from build123d import *

# Parameters (mm, degrees)
SKETCH_1_W           = 135
SKETCH_1_H           = 80
EXTRUDE_1_DEPTH      = 80
SKETCH_6_W           = 45
SKETCH_6_H           = 80
CUT_EXTRUDE_1_DEPTH  = 35
SKETCH_5_W           = 45
SKETCH_5_H           = 80
CUT_EXTRUDE_2_DEPTH  = 35
SKETCH_7_W           = 80
SKETCH_7_H           = 70
CUT_EXTRUDE_3_DEPTH  = 75
SKETCH_8_W           = 87.8
SKETCH_8_H           = 77.8
SKETCH_8_W_2         = 82.2
SKETCH_8_H_2         = 72.2
CUT_EXTRUDE_4_DEPTH  = 10
SKETCH_9_R           = 5
CUT_EXTRUDE_5_DEPTH  = 32.4
SKETCH_10_W          = 21.5
SKETCH_10_H          = 15
CUT_EXTRUDE_6_DEPTH  = 10
SKETCH_12_W          = 15.816906699
SKETCH_12_H          = 10
CUT_EXTRUDE_7_DEPTH  = 45
CUT_EXTRUDE_8_DEPTH  = 3
SKETCH_15_W          = 10
SKETCH_15_H          = 10
CUT_EXTRUDE_9_DEPTH  = 6
SKETCH_17_R          = 1.095275866
CUT_EXTRUDE_11_DEPTH = 7
SKETCH_18_W          = 5
SKETCH_18_H          = 5
SKETCH_18_R          = 1.1
EXTRUDE_2_DEPTH      = 5


with BuildPart() as part:
    # 草圖1 → 填料-伸長1 (new body)
    with BuildSketch(Plane.XY):
        with Locations((-8.008902174, 5.58988764)):
            Rectangle(SKETCH_1_W, SKETCH_1_H)
    extrude(amount=EXTRUDE_1_DEPTH)

    # 草圖6 → 除料-伸長1 (cut)
    with BuildSketch(Plane(origin=(0, 45.58988764, 0), x_dir=(1, 0, 0), z_dir=(0, 1, 0))):
        with Locations((36.991097826, -40)):
            Rectangle(SKETCH_6_W, SKETCH_6_H)
    extrude(amount=-CUT_EXTRUDE_1_DEPTH, mode=Mode.SUBTRACT)

    # 草圖5 → 除料-伸長2 (cut)
    with BuildSketch(Plane.XZ.offset(34.41011236)):
        with Locations((36.991097826, 40)):
            Rectangle(SKETCH_5_W, SKETCH_5_H)
    extrude(amount=-CUT_EXTRUDE_2_DEPTH, mode=Mode.SUBTRACT)

    # 草圖7 → 除料-伸長3 (cut)
    with BuildSketch(Plane.XY):
        with Locations((-30.508902174, 5.58988764)):
            Rectangle(SKETCH_7_W, SKETCH_7_H)
    extrude(amount=CUT_EXTRUDE_3_DEPTH, mode=Mode.SUBTRACT)

    # 草圖8 → 除料-伸長4 (cut)
    with BuildSketch(Plane(origin=(0, 0, 0), x_dir=(-1, 0, 0), z_dir=(0, 0, -1))):
        with Locations((30.508902174, 5.58988764)):
            Rectangle(SKETCH_8_W, SKETCH_8_H)
        with Locations((30.508902174, 5.58988764)):
            Rectangle(SKETCH_8_W_2, SKETCH_8_H_2, mode=Mode.SUBTRACT)
    extrude(amount=-CUT_EXTRUDE_4_DEPTH, mode=Mode.SUBTRACT)

    # 草圖9 → 除料-伸長5 (cut)
    with BuildSketch(Plane(origin=(14.491097826, 0, 0), x_dir=(0, 0, -1), z_dir=(1, 0, 0))):
        with Locations((-65, 30.58988764)):
            Circle(SKETCH_9_R)
        with Locations((-20, -19.41011236)):
            Circle(SKETCH_9_R)
    extrude(amount=-CUT_EXTRUDE_5_DEPTH, mode=Mode.SUBTRACT)

    # 草圖10 → 除料-伸長6 (cut)
    with BuildSketch(Plane(origin=(0, -34.41011236, 0), x_dir=(-1, 0, 0), z_dir=(0, -1, 0))):
        with Locations((24.758902174, -22.5)):
            Rectangle(SKETCH_10_W, SKETCH_10_H)
    extrude(amount=-CUT_EXTRUDE_6_DEPTH, mode=Mode.SUBTRACT)

    # 草圖12 → 除料-伸長7 (cut)
    with BuildSketch(Plane(origin=(14.491097826, 0, 0), x_dir=(0, 0, -1), z_dir=(1, 0, 0))):
        with Locations((-72.09154665, 5.58988764)):
            Rectangle(SKETCH_12_W, SKETCH_12_H)
        with Locations((-7.90845335, 5.58988764)):
            Rectangle(SKETCH_12_W, SKETCH_12_H)
    extrude(amount=CUT_EXTRUDE_7_DEPTH, mode=Mode.SUBTRACT)

    # 草圖14 → 除料-伸長8 (cut)
    with BuildSketch(Plane(origin=(0, 0.58988764, 0), x_dir=(-1, 0, 0), z_dir=(0, -1, 0))):
        with BuildLine():
            Line((-38.009101008, -35.10282789), (-21.517914827, -38.5))
            ThreePointArc((-21.517914827, -38.5), (-20.017914827, -40), (-21.517914827, -41.5))
            Line((-21.517914827, -41.5), (-38.009101008, -44.89717211))
            ThreePointArc((-38.009101008, -44.89717211), (-39.017914827, -45), (-40.026728646, -44.89717211))
            Line((-40.026728646, -44.89717211), (-56.517914827, -41.5))
            ThreePointArc((-56.517914827, -41.5), (-58.017914827, -40), (-56.517914827, -38.5))
            Line((-56.517914827, -38.5), (-40.026728646, -35.10282789))
            ThreePointArc((-40.026728646, -35.10282789), (-39.017914827, -35), (-38.009101008, -35.10282789))
        make_face()
    extrude(amount=-CUT_EXTRUDE_8_DEPTH, mode=Mode.SUBTRACT)

    # 草圖15 → 除料-伸長9 (cut)
    with BuildSketch(Plane(origin=(0, 10.58988764, 0), x_dir=(1, 0, 0), z_dir=(0, 1, 0))):
        with Locations((39.491097826, -39.816906699)):
            Rectangle(SKETCH_15_W, SKETCH_15_H)
    extrude(amount=-CUT_EXTRUDE_9_DEPTH, mode=Mode.SUBTRACT)

    # 草圖17 → 除料-伸長11 (cut)
    with BuildSketch(Plane(origin=(0, 0.58988764, 0), x_dir=(-1, 0, 0), z_dir=(0, -1, 0))):
        with Locations((-39.017914827, -40)):
            Circle(SKETCH_17_R)
    extrude(amount=-CUT_EXTRUDE_11_DEPTH, mode=Mode.SUBTRACT)

    # 草圖18 → 填料-伸長2 (add)
    with BuildSketch(Plane.XY):
        with Locations((11.991097826, 48.08988764)):
            Rectangle(SKETCH_18_W, SKETCH_18_H)
        with Locations((11.991097826, 48.08988764)):
            Circle(SKETCH_18_R, mode=Mode.SUBTRACT)
        with Locations((-73.008902174, 48.08988764)):
            Rectangle(SKETCH_18_W, SKETCH_18_H)
        with Locations((-73.008902174, 48.08988764)):
            Circle(SKETCH_18_R, mode=Mode.SUBTRACT)
        with Locations((-73.008902174, -36.91011236)):
            Rectangle(SKETCH_18_W, SKETCH_18_H)
        with Locations((-73.008902174, -36.91011236)):
            Circle(SKETCH_18_R, mode=Mode.SUBTRACT)
        with Locations((11.991097826, -36.91011236)):
            Rectangle(SKETCH_18_W, SKETCH_18_H)
        with Locations((11.991097826, -36.91011236)):
            Circle(SKETCH_18_R, mode=Mode.SUBTRACT)
    extrude(amount=EXTRUDE_2_DEPTH)


solid = part.part
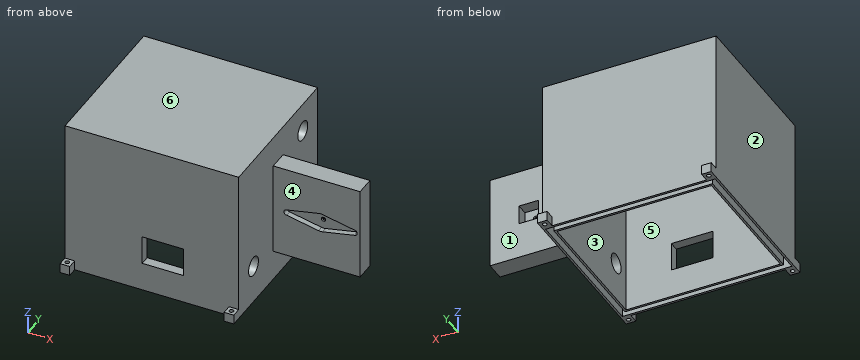
CAD build for the part. Positions are in the model's coordinates, mm. Face numbers are marked on the shaded views. A direction names the side the tool comes from. Round coordinates to 2 decimals unless told otherwise and drop trailing zeros. Order: outer loops, then holes, each group sorted by start corner. A loop starts at its lowest first (then second) coordinate and runs counter-clockwise, first axis right, second up. Notation, with made-up numbers: (-25.5, 57) -> (-17.5, 57) arc R20 ccw to (-17.5, 75) -> close; hole circle Ø8 at (29, 34.25). An arc over 180 degrees is marked (long way). Write item = value, one per line. Start each with the question number.
(1) Cut at D-D, the plane y = 38.5. List the corners of the cut face in (x, z), then the cut area to 3 significant figures.
(2) Cut at C-C, the plane z = 55.5. List the corners of the cut face in (x, y), then the cut area to 3 significant figures.
(3) Pin check, flat tips, straight feed: P1, Ø3.5, axis at x = 11.99, y = 48.09, coming from the -Z side; P2, Ø3, axis at x = -32.5, z = 50.5, coming from the +Y side; P3, Ø4, axis at x = -44.5, y = -25.5, coming from the -Z side; P4, Ø11, axis at x = 43.5, z = 38, coming from the -Y side. Stop position of each tip, or through.
(4) Cut at B-B, the plane z = 20. List the corners of the cut face in (x, y), then the cut area to 3 significant figures.
(5) Probe line 1 (Y direction, x = -70, z = 22); line 2 (X direction, y = -21.5, z = 65); line 3 (X direction, y = -29.5, z = 21). List the from-to ranges inside material, lowest first. Write a range as [from, to].
(6) Which spindle directions (+Z, -Z, +X, -X, +Y, -Y) get a long thin tool onto all of the face, cutting with end or side? Do the marked faces 4, 5 and 6. Say none if no direction does.
(7) Cut at A-A, the plane x = -20.5. List the corners of the cut face in (y, z).
(8) Pull direction Y, two halves, no side cores. Call the marked faces 1, 2 and 3: released by +Y, released by -Y, zero draft, split by the parting line, or undercut.
Model answer:
q1.outline = (-75.51, 0) -> (-74.41, 0) -> (-74.41, 10) -> (-71.61, 10) -> (-71.61, 0) -> (-70.51, 0) -> (-70.51, 75) -> (9.49, 75) -> (9.49, 0) -> (10.59, 0) -> (10.59, 10) -> (13.39, 10) -> (13.39, 0) -> (14.49, 0) -> (14.49, 80) -> (-75.51, 80) -> close
q1.area = 1,140 mm2
q2.outline = (-75.51, -34.41) -> (14.49, -34.41) -> (14.49, 0.59) -> (59.49, 0.59) -> (59.49, 10.59) -> (14.49, 10.59) -> (14.49, 45.59) -> (-75.51, 45.59) -> close; hole (-70.51, -29.41) -> (9.49, -29.41) -> (9.49, 40.59) -> (-70.51, 40.59) -> close
q2.area = 2,050 mm2
q3.P1 = 0
q3.P2 = 45.59
q3.P3 = 75
q3.P4 = 0.59
q4.outline = (-75.51, -34.41) -> (-35.51, -34.41) -> (-35.51, -29.41) -> (-70.51, -29.41) -> (-70.51, 40.59) -> (9.49, 40.59) -> (9.49, -14.41) -> (14.49, -14.41) -> (14.49, 0.59) -> (59.49, 0.59) -> (59.49, 10.59) -> (14.49, 10.59) -> (14.49, 45.59) -> (-75.51, 45.59) -> close; (-14.01, -34.41) -> (14.49, -34.41) -> (14.49, -24.41) -> (9.49, -24.41) -> (9.49, -29.41) -> (-14.01, -29.41) -> close
q4.area = 1,890 mm2
q5.line_1 = [-34.41, -29.41], [40.59, 45.59]
q5.line_2 = [-75.51, -70.51], [9.49, 14.49]
q5.line_3 = [-75.51, -35.51], [-14.01, 14.49]
q6.face_4 = +Z, -Z, +X, -Y
q6.face_5 = -Z
q6.face_6 = +Z, +X, -X, +Y, -Y
q7.outline = (-34.41, 0) -> (-33.31, 0) -> (-33.31, 10) -> (-30.51, 10) -> (-30.51, 0) -> (-29.41, 0) -> (-29.41, 15) -> (-34.41, 15) -> close; (-34.41, 30) -> (-29.41, 30) -> (-29.41, 75) -> (40.59, 75) -> (40.59, 0) -> (41.69, 0) -> (41.69, 10) -> (44.49, 10) -> (44.49, 0) -> (45.59, 0) -> (45.59, 80) -> (-34.41, 80) -> close
q8.face_1 = released by +Y
q8.face_2 = zero draft
q8.face_3 = undercut
